from build123d import *

# Parameters (mm, degrees)
F0_W     = 12
F0_H     = 12
F1_DEPTH = 8


with BuildPart() as f1:
    # F0 (on Top) → F1 (new body)
    with BuildSketch(Plane.XY):
        Polygon((-187.250624, 322.639689), (-227.250624, 322.639689), (-227.250624, -151.360311), (-223.250624, -151.360311), (-223.250624, -163.360311), (-227.250624, -163.360311), (-227.250624, -177.360311), (224.749376, -177.360311), (224.749376, 347.639689), (184.749376, 347.639689), (184.749376, -137.360311), (-1.250624, -137.360311), (-187.250624, -137.360311), align=None)
        with Locations((-115.250624, -157.360311)):
            Rectangle(F0_W, F0_H, mode=Mode.SUBTRACT)
        Polygon((-7.250624, -151.360311), (-1.250624, -151.360311), (4.749376, -151.360311), (4.749376, -163.360311), (-7.250624, -163.360311), align=None, mode=Mode.SUBTRACT)
        with Locations((112.749376, -157.360311)):
            Rectangle(F0_W, F0_H, mode=Mode.SUBTRACT)
    extrude(amount=F1_DEPTH)


solid = f1.part
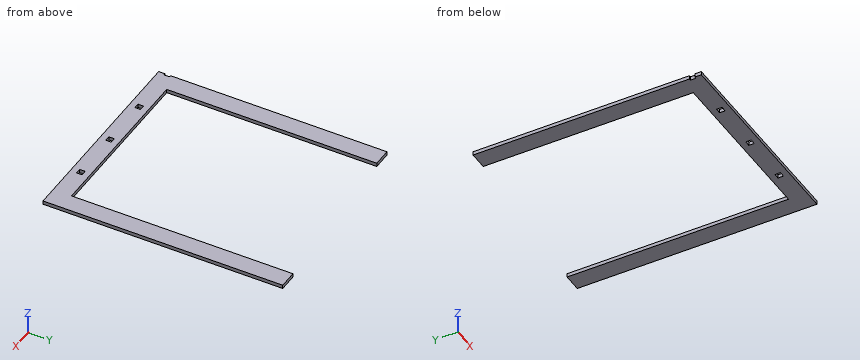
The listing builds one solid part. Answer for the finished solid, in the listing's coordinates (mm). Round coordinates to 2 decimals unless told otherwise and drop trailing zeros. Write each loop counter-clockwise with the first axis right and the second up, starting at its lowest first coordinate (ties: lowest second). Pieces come first, ordered by that corner, then holes. Notation, with made-up numbers: (8.5, 36) - (17.5, 36) arc R27 cw to (17.5, 58) - close; hole circle Ø11 at (57.5, -27.5). An arc over 180 degrees is marked (long way). Use one line per item in the form item = value. Start each with the question number.
Item 1: A cutting plane is placed at C-C (x = -193). Write down the section's boundary in (y, z).
Item 2: Find the intervals of material crossed by line 1 (X direction, y = -94, z = 0.5); line 2 (Y direction, x = -188.5, z = 6); line 3 (Y direction, x = -55.5, z = 0.5), in increasing order. Write a range as [from, to].
Item 3: Flat-ended cylindrical pins translate along their axes: pin 1 Ø4 at (y, z) = (-155.5, 2.5) entering from -X; pin 2 Ø1.5 at (x, z) = (-169.5, 4.5) entering from +Y; pin 3 Ø2 at (x, z) = (-226, 3) entering from +Y. Find the tip coordinate at first contact, or state that the pin passes through.
Item 4: A cutting plane is placed at B-B (z = 2). Write down the section's boundary in (x, y).
Item 5: A cutting plane is placed at D-D (x = 79.5). Write down the section's boundary in (y, z).
Item 6: A cutting plane is placed at A-A (y = 269). Write down the section's boundary in (x, z), plus the area to 3 significant figures.
The answers:
q1.outline = (-177.36, 0) - (322.64, 0) - (322.64, 8) - (-177.36, 8) - close
q2.line_1 = [-227.25, -187.25], [184.75, 224.75]
q2.line_2 = [-177.36, 322.64]
q2.line_3 = [-177.36, -137.36]
q3.pin_1 = -223.25
q3.pin_2 = -137.36
q3.pin_3 = 322.64
q4.outline = (-227.25, -177.36) - (224.75, -177.36) - (224.75, 347.64) - (184.75, 347.64) - (184.75, -137.36) - (-187.25, -137.36) - (-187.25, 322.64) - (-227.25, 322.64) - (-227.25, -151.36) - (-223.25, -151.36) - (-223.25, -163.36) - (-227.25, -163.36) - close; hole (-121.25, -163.36) - (-109.25, -163.36) - (-109.25, -151.36) - (-121.25, -151.36) - close; hole (-7.25, -163.36) - (4.75, -163.36) - (4.75, -151.36) - (-7.25, -151.36) - close; hole (106.75, -163.36) - (118.75, -163.36) - (118.75, -151.36) - (106.75, -151.36) - close
q5.outline = (-177.36, 0) - (-137.36, 0) - (-137.36, 8) - (-177.36, 8) - close
q6.outline = (-227.25, 0) - (-187.25, 0) - (-187.25, 8) - (-227.25, 8) - close; (184.75, 0) - (224.75, 0) - (224.75, 8) - (184.75, 8) - close
q6.area = 640 mm^2
